Verification items for the finished model (mm, model axes). A direction names the side the tool comes from. Coordinates: 2 decimals unless noted, no trailing zeros. Write each loop counter-clockwise with the first axis right and the second up, starting at its lowest first coordinate (ties: lowest second). Pieces come first, ordered by that corner, then holes. Notation, with made-up numbers: (23.25, -28.75) -> (44.25, -28.75) arc R24 ccw to (44.25, -12.75) -> close; hole circle Ø9 at (34, 1.25). An arc over 180 degrees is marked (long way). Use a Markdown table: item, result. Add a question column.
from build123d import *

# Parameters (mm, degrees)
F1_DEPTH       = 20
F2_W           = 12.5
F2_H           = 30
F3_DEPTH       = 7
F4_DEPTH       = 3
F7_D           = 6.6
F7_DEPTH       = 15.001
F7_ON_F5_D     = 6.6
F7_ON_F5_DEPTH = 15.001
F9_D           = 5


with BuildPart() as f1:
    # F0 (on Top) → F1 (new body)
    with BuildSketch(Plane.XY):
        Polygon((37.5, 35.5), (-37.5, 35.5), (-37.5, 20.5), (-17.5, 20.5), (-17.5, 0), (-17.5, -20.5), (-37.5, -20.5), (-37.5, -35.5), (37.5, -35.5), (37.5, -20.5), (17.5, -20.5), (17.5, 0), (17.5, 20.5), (37.5, 20.5), align=None)
    extrude(amount=F1_DEPTH)

    # F2 (on face) → F3 (cut)
    with BuildSketch(Plane.XY.offset(20)):
        with Locations((-6.25, 15)):
            Rectangle(F2_W, F2_H)
        Polygon((0, 30), (0, 0), (-12.5, 0), (-12.5, -30), (0, -30), (12.5, -30), (12.5, 0), (12.5, 30), align=None)
    extrude(amount=-F3_DEPTH, mode=Mode.SUBTRACT)

    # F2 (on face) → F4 (cut)
    with BuildSketch(Plane.XY.offset(20)):
        Polygon((-12.5, -30), (-12.5, 0), (-12.5, 30), (-37.5, 30), (-37.5, 20.5), (-17.5, 20.5), (-17.5, -20.5), (-37.5, -20.5), (-37.5, -30), align=None)
    extrude(amount=-F4_DEPTH, mode=Mode.SUBTRACT)

    # F7 (through all, one way)
    with BuildSketch(Plane(origin=(0, -20.5, 0), x_dir=(-1, 0, 0), z_dir=(0, 1, 0))):
        with Locations((27.5, 10), (-27.5, 10)):
            Circle(F7_D / 2)
    extrude(amount=-F7_DEPTH, mode=Mode.SUBTRACT)

    # F7 on F5 (through all, one way)
    with BuildSketch(Plane.XZ.offset(-20.5)):
        with Locations((-27.5, 10), (27.5, 10)):
            Circle(F7_ON_F5_D / 2)
    extrude(amount=-F7_ON_F5_DEPTH, mode=Mode.SUBTRACT)

    # F9 (through all)
    with Locations(Plane.XY.offset(20)):
        with Locations((-6.5, 23), (6.5, 23), (6.5, -23), (-6.5, -23)):
            Hole(F9_D / 2)


solid = f1.part
1) Cross-section at A-A on y = -23. Record the boundary of the cut face in (x, z).
2) Set-up check for faces 1 (the face through (-12.5, 0, 15)), 2 (the face through (-17.5, 0, 8)), 3 (the face through (-24.45, 27.9, 8.74)), 4 (the face through (23, 20.5, 10)): record each of +Z, -Z, +X, -X, +Y, -Y from which the full face is reachable in a straight line by a thin tool's end or side.
3) Gauge pin test, flat ends, axial feed: pin 1 (5 mm diameter, centred on y = 9, z = 7, fed in from +X); pin 2 (2 mm diameter, centred on y = 4.5, z = 4.5, fed in from -X); pin 3 (7.5 mm diameter, centred on x = 4, y = -0.5, fed in from +Z). Record the tip position at first contact, or that the pin passes through.
4) Release check for a two-part mould opening along X. For faces 5 (the face through (17.5, 0, 10)), 6 (the face through (1, 35.5, 10)), 7 (the face through (-7, 30, 17)) record: released by +X, released by -X, zero draft, split by the parting line, or undercut.
5) Cross-section at B-B on x = -27.5. Record the boundary of the cut face in (y, z), then the cut area to 3 significant figures.
6) Thickness scan on L1, parallel to Y at x = -6.5, z = 2.75; L2, parallel to Y at x = -13, z = 18.75; L3, parallel to Y at x = -23, z = 9.5. Record the ranges inside material, lowest first.
7) Cross-section at C-C on z = 15. Record the boundary of the cut face in (x, y).
8) Cross-section at D-D on x = 6.5. Record the boundary of the cut face in (y, z), then the cut area to 3 significant figures.
Returned:
| question | item | result |
|---|---|---|
| 1 | outline | (-37.5, 0) -> (-9, 0) -> (-9, 13) -> (-12.5, 13) -> (-12.5, 17) -> (-37.5, 17) -> close; (-4, 0) -> (4, 0) -> (4, 13) -> (-4, 13) -> close; (9, 0) -> (37.5, 0) -> (37.5, 20) -> (12.5, 20) -> (12.5, 13) -> (9, 13) -> close; hole circle Ø6.6 at (-27.5, 10); hole circle Ø6.6 at (27.5, 10) |
| 2 | face 1 | +Z |
| 2 | face 2 | +Z, -Z, -X |
| 2 | face 3 | +Y, -Y |
| 2 | face 4 | +Z, -Z, +X |
| 3 | pin 1 | stops at x = 17.5 |
| 3 | pin 2 | stops at x = -17.5 |
| 3 | pin 3 | stops at z = 13 |
| 4 | face 5 | released by +X |
| 4 | face 6 | zero draft |
| 4 | face 7 | undercut |
| 5 | outline | (-35.5, 0) -> (-20.5, 0) -> (-20.5, 6.7) -> (-35.5, 6.7) -> close; (-35.5, 13.3) -> (-20.5, 13.3) -> (-20.5, 17) -> (-30, 17) -> (-30, 20) -> (-35.5, 20) -> close; (20.5, 0) -> (35.5, 0) -> (35.5, 6.7) -> (20.5, 6.7) -> close; (20.5, 13.3) -> (35.5, 13.3) -> (35.5, 20) -> (30, 20) -> (30, 17) -> (20.5, 17) -> close |
| 5 | area | 345 mm² |
| 6 | L1 | y = -35.5 to -25.5, -20.5 to 20.5, 25.5 to 35.5 |
| 6 | L2 | y = -35.5 to -30, 30 to 35.5 |
| 6 | L3 | y = -35.5 to -20.5, 20.5 to 35.5 |
| 7 | outline | (-37.5, -35.5) -> (37.5, -35.5) -> (37.5, -20.5) -> (17.5, -20.5) -> (17.5, 20.5) -> (37.5, 20.5) -> (37.5, 35.5) -> (-37.5, 35.5) -> (-37.5, 20.5) -> (-17.5, 20.5) -> (-17.5, -20.5) -> (-37.5, -20.5) -> close; hole (-12.5, -30) -> (12.5, -30) -> (12.5, 30) -> (-12.5, 30) -> close |
| 8 | outline | (-35.5, 0) -> (-25.5, 0) -> (-25.5, 13) -> (-30, 13) -> (-30, 20) -> (-35.5, 20) -> close; (-20.5, 0) -> (20.5, 0) -> (20.5, 13) -> (-20.5, 13) -> close; (25.5, 0) -> (35.5, 0) -> (35.5, 20) -> (30, 20) -> (30, 13) -> (25.5, 13) -> close |
| 8 | area | 870 mm² |
